from build123d import *

# Parameters (mm, degrees)
SKETCH_1_R           = 20
SKETCH_1_W           = 48
SKETCH_1_H           = 7
EXTRUDE_1_DEPTH      = 5
SKETCH_3_R           = 1.75
CUT_EXTRUDE_1_DEPTH  = 11
EXTRUDE_3_DEPTH      = 5
FILLET_8_R           = 2
FILLET_9_R           = 7
FILLET_10_R          = 10
SKETCH_9_R           = 1.75
CUT_EXTRUDE_2_DEPTH  = 5
EXTRUDE_START        = 15
SKETCH_10_R          = 1.75
EXTRUDE_4_DEPTH      = 15
CUT_EXTRUDE_4_DEPTH  = 40
FILLET_11_R          = 5
FILLET_12_R          = 10
FILLET_13_R          = 10
FILLET_14_R          = 5
SKETCH_17_R          = 7.5
CUT_EXTRUDE_9_DEPTH  = 10
SKETCH_18_R          = 12.5
CUT_EXTRUDE_10_DEPTH = 10
SKETCH_21_R          = 1.5
CUT_EXTRUDE_13_DEPTH = 10


with BuildPart() as part:
    # 草图1 → 凸台-拉伸1 (new body)
    with BuildSketch(Plane(origin=(0, 0, 0), x_dir=(1, 0, 0), z_dir=(0, 1, 0))):
        Circle(SKETCH_1_R)
        with BuildLine():
            Line((95, 20), (0, 20))
            ThreePointArc((0, 20), (14.142135624, 14.142135624), (20, 0))
            ThreePointArc((20, 0), (14.142135624, -14.142135624), (0, -20))
            Line((0, -20), (47, -20))
            Line((47, -20), (95, -20))
            Line((95, -20), (95, 20))
        make_face()
        with Locations((71, -23.5)):
            Rectangle(SKETCH_1_W, SKETCH_1_H)
    extrude(amount=EXTRUDE_1_DEPTH)

    # 草图3 → 切除-拉伸1 (cut)
    with BuildSketch(Plane(origin=(0, 5, 0), x_dir=(1, 0, 0), z_dir=(0, 1, 0))):
        with Locations(Location((0, 13.5, 0), (0, 0, 270))):
            Circle(SKETCH_3_R)
        with Locations(Location((11.691342951, 6.75, 0), (0, 0, 270))):
            Circle(SKETCH_3_R)
        with Locations(Location((11.691342951, -6.75, 0), (0, 0, 270))):
            Circle(SKETCH_3_R)
        with Locations(Location((0, -13.5, 0), (0, 0, 270))):
            Circle(SKETCH_3_R)
        with Locations(Location((-11.691342951, -6.75, 0), (0, 0, 270))):
            Circle(SKETCH_3_R)
        with Locations(Location((-11.691342951, 6.75, 0), (0, 0, 270))):
            Circle(SKETCH_3_R)
    extrude(amount=-CUT_EXTRUDE_1_DEPTH, mode=Mode.SUBTRACT)

    # 草图8 → 凸台-拉伸3 (add)
    with BuildSketch(Plane.XY.offset(27)):
        with BuildLine():
            Line((95, 46.8), (95, 0))
            Line((95, 0), (47, 0))
            Line((47, 0), (47, 46.8))
            ThreePointArc((47, 46.8), (71, 70.8), (95, 46.8))
        make_face()
    extrude(amount=-EXTRUDE_3_DEPTH)

    # 圆角8
    fillet_8_edges = [part.edges().sort_by_distance(p)[0] for p in [
        (71, 5, 22),
    ]]
    fillet(fillet_8_edges, radius=FILLET_8_R)

    # 圆角9
    fillet_9_edges = [part.edges().sort_by_distance(p)[0] for p in [
        (71, 0, 27),
    ]]
    fillet(fillet_9_edges, radius=FILLET_9_R)

    # 圆角10
    fillet_10_edges = [part.edges().sort_by_distance(p)[0] for p in [
        (95, 2.5, -20),
    ]]
    fillet(fillet_10_edges, radius=FILLET_10_R)

    # 草图9 → 切除-拉伸2 (cut)
    with BuildSketch(Plane.XY.offset(27)):
        with Locations((57.564971157, 60.235028843)):
            Circle(SKETCH_9_R)
        with Locations((84.435028843, 60.235028843)):
            Circle(SKETCH_9_R)
        with Locations((84.435028843, 33.364971157)):
            Circle(SKETCH_9_R)
        with Locations((57.564971157, 33.364971157)):
            Circle(SKETCH_9_R)
    extrude(amount=-CUT_EXTRUDE_2_DEPTH, mode=Mode.SUBTRACT)

    # 草图10 → 凸台-拉伸4 (add)
    with BuildSketch(Plane(origin=(0, 5, 0), x_dir=(1, 0, 0), z_dir=(0, 1, 0)).offset(EXTRUDE_START)):
        with BuildLine():
            Line((50, 20), (0, 20))
            ThreePointArc((0, 20), (-20, -7e-09), (1.4e-08, -20))
            Line((1.4e-08, -20), (50, -20))
            Line((50, -20), (50, 20))
        make_face()
        with Locations(Location((11.691342951, 6.75, 0), (0, 0, 270))):
            Circle(SKETCH_10_R, mode=Mode.SUBTRACT)
        with Locations(Location((0, 13.5, 0), (0, 0, 270))):
            Circle(SKETCH_10_R, mode=Mode.SUBTRACT)
        with Locations(Location((0, -13.5, 0), (0, 0, 270))):
            Circle(SKETCH_10_R, mode=Mode.SUBTRACT)
        with Locations(Location((-11.691342951, -6.75, 0), (0, 0, 270))):
            Circle(SKETCH_10_R, mode=Mode.SUBTRACT)
        with Locations(Location((11.691342951, -6.75, 0), (0, 0, 270))):
            Circle(SKETCH_10_R, mode=Mode.SUBTRACT)
        with Locations(Location((-11.691342951, 6.75, 0), (0, 0, 270))):
            Circle(SKETCH_10_R, mode=Mode.SUBTRACT)
    extrude(amount=-EXTRUDE_4_DEPTH)

    # 草图11 → 切除-拉伸4 (cut)
    with BuildSketch(Plane(origin=(0, 0, -20), x_dir=(-1, 0, 0), z_dir=(0, 0, -1))):
        Polygon((-50, 5), (-37, 5), (-22, 20), (-50, 20), align=None)
        Polygon((20, 0), (20, 15), (-19.928932188, 15), (-34.928932188, 0), align=None)
    extrude(amount=-CUT_EXTRUDE_4_DEPTH, mode=Mode.SUBTRACT)

    # 圆角11
    fillet_11_edges = [part.edges().sort_by_distance(p)[0] for p in [
        (19.928932188, 15, 0),
    ]]
    fillet(fillet_11_edges, radius=FILLET_11_R)

    # 圆角12
    fillet_12_edges = [part.edges().sort_by_distance(p)[0] for p in [
        (22, 20, 0),
    ]]
    fillet(fillet_12_edges, radius=FILLET_12_R)

    # 圆角13
    fillet_13_edges = [part.edges().sort_by_distance(p)[0] for p in [
        (34.928932188, 0, 0),
    ]]
    fillet(fillet_13_edges, radius=FILLET_13_R)

    # 圆角14
    fillet_14_edges = [part.edges().sort_by_distance(p)[0] for p in [
        (37, 5, 0),
    ]]
    fillet(fillet_14_edges, radius=FILLET_14_R)

    # 草图17 → 切除-拉伸9 (cut)
    with BuildSketch(Plane(origin=(0, 20, 0), x_dir=(1, 0, 0), z_dir=(0, 1, 0))):
        with Locations(Location((0, 0, 0), (0, 0, 270))):
            Circle(SKETCH_17_R)
    extrude(amount=-CUT_EXTRUDE_9_DEPTH, mode=Mode.SUBTRACT)

    # 草图18 → 切除-拉伸10 (cut)
    with BuildSketch(Plane.XY.offset(27)):
        with Locations((71, 46.8)):
            Circle(SKETCH_18_R)
    extrude(amount=-CUT_EXTRUDE_10_DEPTH, mode=Mode.SUBTRACT)

    # 草图21 → 切除-拉伸13 (cut)
    with BuildSketch(Plane.XZ):
        with Locations(Location((87, 12, 0), (0, 0, 270))):
            Circle(SKETCH_21_R)
        with Locations(Location((47.071067812, -12, 0), (0, 0, 270))):
            Circle(SKETCH_21_R)
        with Locations(Location((47.071067812, 12, 0), (0, 0, 270))):
            Circle(SKETCH_21_R)
        with Locations(Location((87, -12, 0), (0, 0, 270))):
            Circle(SKETCH_21_R)
    extrude(amount=-CUT_EXTRUDE_13_DEPTH, mode=Mode.SUBTRACT)


solid = part.part
Build history of the part. All positions in model axes, mm. A direction names the side the tool comes from. Give positions to 0.01 mm unless a question says otherwise; leave off trailing zeros. Loops run counter-clockwise (first coordinate to the right, second up) from the corner with the lowest first, then second, coordinate; pieces in that order, holes last. Notation, with made-up numbers: (43, 66.25) -> (60, 66.25) arc R30 ccw to (60, 105.25) -> close; hole circle Ø10 at (42, -18.75). An arc over 180 degrees is marked (long way). Answer in a Markdown table with one row per item.
Item 1: Slice it at B-B on y = 39.5. Write the cut outline in (x, z).
Findings below:
| item | result |
|---|---|
| outline | (47, 22) -> (60.85, 22) -> (60.85, 27) -> (47, 27) -> close; (81.15, 22) -> (95, 22) -> (95, 27) -> (81.15, 27) -> close |
Item 2: Slice it at A-A on x = 71. Write the cut outline in (y, z).
Findings below:
| item | result |
|---|---|
| outline | (0, -20) -> (5, -20) -> (5, 20) arc R2 cw to (7, 22) -> (34.3, 22) -> (34.3, 27) -> (7, 27) arc R7 ccw to (0, 20) -> close; (59.3, 22) -> (70.8, 22) -> (70.8, 27) -> (59.3, 27) -> close |
Item 3: Tool access for faces 1 (the flat face through (7, 15, 4)), 2 (the cylindrical face through (37.18, 5.37, 0.28)): list every direction of +Z, -Z, +X, -X, +Y, -Y with a clear straight run to the whole face (end or side of a thin tool).
Findings below:
| item | result |
|---|---|
| face 1 | +Z, -Z, -X, -Y |
| face 2 | +Z, -Z, +X, +Y |
Item 4: Mould opens along X. For faces 3 (the cylindrical face through (35.193, 0.782, 0.28)), 4 (the cylindrical face through (57.186, 58.527, 24.535)), 5 (the flat face through (71, 32, 22)), 6 (the cylindrical face through (70.472, 70.794, 24.535)) say: pulls with the +X half, pulls with the -X half, needs draft (parallel to the pull), parting line crosses it, or undercut.
Findings below:
| item | result |
|---|---|
| face 3 | pulls with the -X half |
| face 4 | undercut |
| face 5 | needs draft |
| face 6 | parting line crosses it |
Item 5: Probe line 1 along X through (y, z) = (3.85, -12); line 2 along Y through (x, z) = (75, -1.5); line 3 along X through (y, z) = (10, 18). List the from-to ranges inside material, lowest first. Write a range as [from, to].
Findings below:
| item | result |
|---|---|
| line 1 | x = [31.08, 45.57], [48.57, 85.5], [88.5, 94.8] |
| line 2 | y = [0, 5] |
| line 3 | x = [24.93, 32] |
Item 6: Flat gauge pins, fed straight in: P1, Ø5.5, axis at x = 0, z = -13.5, coming from the +Y side; P2, Ø17, axis at x = 0, z = 0, coming from the -Y side; P3, Ø5, axis at y = 14, z = -10.5, coming from the -X side. Where does each tip first touch, or does it go through?
Findings below:
| item | result |
|---|---|
| P1 | stops at y = 20 |
| P2 | stops at y = 15 |
| P3 | stops at x = -18.24 |
Item 7: Slice it at D-D on x = 29. Write the cut outline in (y, z).
Findings below:
| item | result |
|---|---|
| outline | (5.93, -20) -> (13, -20) -> (13, 20) -> (5.93, 20) -> close |
Item 8: Slice it at C-C on y = 28.5. Write the cut outline in (x, z), plus the area to 3 significant figures.
Findings below:
| item | result |
|---|---|
| outline | (47, 22) -> (95, 22) -> (95, 27) -> (47, 27) -> close |
| area | 240 mm² |
